from build123d import *

# Parameters (mm, degrees)
BOSS_EXTRUDE1_DEPTH = 0.5
SKETCH2_R           = 1
CUT_EXTRUDE1_DEPTH  = 11.9573035
FILLET1_R           = 0.2


with BuildPart() as part:
    # Sketch1 → Boss-Extrude1 (new, symmetric)
    with BuildSketch(Plane.XY):
        with BuildLine():
            Line((-5.661803514, 6.995997497), (-6.226216863, 0.544723392))
            ThreePointArc((-6.226216863, 0.544723392), (0, -6.25), (6.226216863, 0.544723392))
            Line((6.226216863, 0.544723392), (5.661803514, 6.995997497))
            ThreePointArc((5.661803514, 6.995997497), (3.470425019, 8.303983995), (1, 8.94427191))
            Line((1, 8.94427191), (1, 4.643543905))
            ThreePointArc((1, 4.643543905), (0, -4.75), (-1, 4.643543905))
            Line((-1, 4.643543905), (-1, 8.94427191))
            ThreePointArc((-1, 8.94427191), (-3.470425019, 8.303983995), (-5.661803514, 6.995997497))
        make_face()
    extrude(amount=BOSS_EXTRUDE1_DEPTH, both=True)

    # Sketch2 → Cut-Extrude1 (cut, through all)
    with BuildSketch(Plane.XY.offset(0.5)):
        with Locations((-3.605551275, 6)):
            Circle(SKETCH2_R)
        with Locations((3.605551275, 6)):
            Circle(SKETCH2_R)
    extrude(amount=-CUT_EXTRUDE1_DEPTH, mode=Mode.SUBTRACT)

    # Fillet1
    fillet1_edges = [part.edges().sort_by_distance(p)[0] for p in [
        (5.661803514, 6.995997497, 0),
        (-5.661803514, 6.995997497, 0),
        (-1, 8.94427191, 0),
        (-1, 4.643543905, 0),
        (1, 4.643543905, 0),
        (1, 8.94427191, 0),
    ]]
    fillet(fillet1_edges, radius=FILLET1_R)


solid = part.part
Here's how the part is built. I have some questions about the finished solid (model axes, mm). A direction names the side the tool comes from. Coordinates: 2 decimals unless noted, no trailing zeros. Loops run counter-clockwise (first coordinate to the right, second up) from the corner with the lowest first, then second, coordinate; pieces in that order, holes last.
1. If we mould it in two halves opening along Y, with no side actions, what happens to faces 1 (the cylindrical face through (0.193, -4.746, 0.007)), 2 (the flat face through (-5.944, 3.772, 0.007)), 3 (the cylindrical face through (4.143, 6.843, 0.007)), 4 (the flat face through (1.3, 4.8, 0.5))? For each: pulls with the +Y half, pulls with the -Y half, needs draft (parallel to the pull), parting line crosses it, or undercut.
2. Imagine slicing it at A-A, the plane z = 0.2. Please give me the cut outline in (x, y).
3. Imagine slicing it at B-B, the plane y = 0. Please give me the cut outline in (x, z).
4. I need wall thicknesses on L1, parallel to Y at x = 3.75, z = 0.05; L2, parallel to X at y = 0, z = -0.2; L3, parallel to X at y = 3.5, z = -0.3. Which ranges of each line are inside material? Lowest first, please.
5. For P1, Ø1, axis at x = 4, y = 0.5, coming from the +Z side; P2, Ø0.5, axis at y = 6.5, z = 0, coming from the -X side, each with a flat end and sliding along its axis, tell me the tip position at first contact or that it passes through.
6. For faces 5 (the flat face through (1, 7, 0)), 6 (the cylindrical face through (-4.34, 6.68, 0.01)), which set-ups out of +Z, -Z, +X, -X, +Y, -Y let a thin tool reach every point of the face, with its end or its side?
7. Imagine slicing it at C-C, the plane x = 1.75. Please give me the cut outline in (y, z).
8. Imagine slicing it at D-D, the plane y = 6. Please give me the cut outline in (x, z).
Taken from the geometry:
1. face 1: undercut
1. face 2: pulls with the +Y half
1. face 3: undercut
1. face 4: needs draft
2. outline: (-6.23, 0.54) arc R6.25 ccw (long way) to (6.23, 0.54) - (5.67, 6.91) arc R0.2 ccw to (5.59, 7.05) arc R9 ccw to (1.23, 8.92) arc R0.2 ccw to (1, 8.72) - (1, 4.8) arc R0.2 ccw to (1.15, 4.61) arc R4.75 cw (long way) to (-1.15, 4.61) arc R0.2 ccw to (-1, 4.8) - (-1, 8.72) arc R0.2 ccw to (-1.23, 8.92) arc R9 ccw to (-5.59, 7.05) arc R0.2 ccw to (-5.67, 6.91) - close; hole circle Ø2 at (-3.61, 6); hole circle Ø2 at (3.61, 6)
3. outline: (-6.25, -0.5) - (-4.75, -0.5) - (-4.75, 0.5) - (-6.25, 0.5) - close; (4.75, -0.5) - (6.25, -0.5) - (6.25, 0.5) - (4.75, 0.5) - close
4. L1: y = -5 to -2.92, 2.92 to 5.01, 6.99 to 8.18
4. L2: x = -6.25 to -4.75, 4.75 to 6.25
4. L3: x = -5.97 to -3.21, 3.21 to 5.97
5. P1: passes through
5. P2: stops at x = -5.73
6. face 5: +Z, -Z, +Y
6. face 6: +Z, -Z
7. outline: (-6, -0.5) - (-4.42, -0.5) - (-4.42, 0.5) - (-6, 0.5) - close; (4.42, -0.5) - (8.83, -0.5) - (8.83, 0.5) - (4.42, 0.5) - close
8. outline: (-5.75, -0.5) - (-4.61, -0.5) - (-4.61, 0.5) - (-5.75, 0.5) - close; (-2.61, -0.5) - (-1, -0.5) - (-1, 0.5) - (-2.61, 0.5) - close; (1, -0.5) - (2.61, -0.5) - (2.61, 0.5) - (1, 0.5) - close; (4.61, -0.5) - (5.75, -0.5) - (5.75, 0.5) - (4.61, 0.5) - close
